from build123d import *

# Parameters (mm, degrees)
F1_DEPTH = 5
F0_W     = 6
F0_H     = 5.5
F0_R     = 1.5
F0_H_2   = 5.75
F2_DEPTH = 25
F4_DEPTH = 105


with BuildPart() as f1:
    # F0 (on Top) → F1 (new body)
    with BuildSketch(Plane.XY):
        Polygon((43.5, 30.25), (-43.5, 30.25), (-43.5, 24.75), (-49.5, 24.75), (-49.5, -24.5), (-43.5, -24.5), (-43.5, -30.25), (43.5, -30.25), (43.5, -24.5), (49.5, -24.5), (49.5, 24.5), (43.5, 24.5), align=None)
    extrude(amount=F1_DEPTH)

    # F0 (on Top) → F2 (join)
    with BuildSketch(Plane.XY):
        with Locations((-46.5, 27.5)):
            Rectangle(F0_W, F0_H)
        with Locations((-46.5, 27.5)):
            Circle(F0_R, mode=Mode.SUBTRACT)
        with Locations((-46.5, -27.375)):
            Rectangle(F0_W, F0_H_2)
        with Locations((-46.5, -27.5)):
            Circle(F0_R, mode=Mode.SUBTRACT)
        with Locations((46.5, -27.375)):
            Rectangle(F0_W, F0_H_2)
        with Locations((46.5, -27.5)):
            Circle(F0_R, mode=Mode.SUBTRACT)
        with Locations((46.5, 27.375)):
            Rectangle(F0_W, F0_H_2)
        with Locations((46.5, 27.5)):
            Circle(F0_R, mode=Mode.SUBTRACT)
    extrude(amount=F2_DEPTH)

    # F3 (on face) → F4 (cut)
    with BuildSketch(Plane.YZ.offset(49.5)):
        Polygon((34.920923, 25), (34.537785, 31.615168), (-33.879854, 31.615168), (-33.879854, 17.220095), align=None)
    extrude(amount=-F4_DEPTH, mode=Mode.SUBTRACT)


solid = f1.part
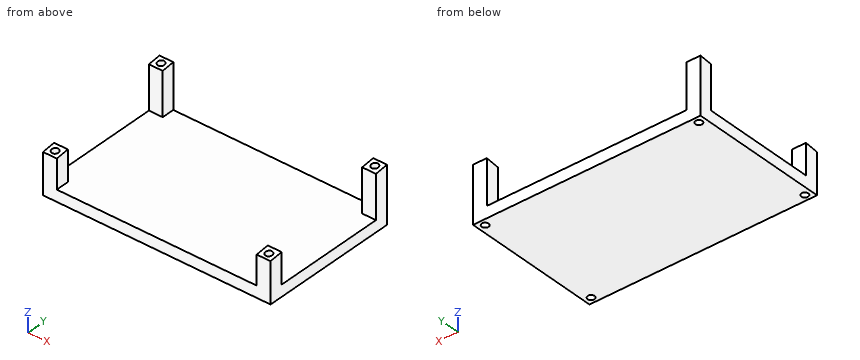
Verification items for the finished model (mm, model axes). Give positions to 0.01 mm unless a question says otherwise; leave off trailing zeros. Loops run counter-clockwise (first coordinate to the right, second up) from the corner with the lowest first, then second, coordinate; pieces in that order, holes last.
1. Cross-section at B-B on z = 8.25. Record the cut outline in (x, y), and give its area (3 significant figures).
Derived:
outline: (-49.5, -30.25) - (-43.5, -30.25) - (-43.5, -24.5) - (-49.5, -24.5) - close; (-49.5, 24.75) - (-43.5, 24.75) - (-43.5, 30.25) - (-49.5, 30.25) - close; (43.5, -30.25) - (49.5, -30.25) - (49.5, -24.5) - (43.5, -24.5) - close; (43.5, 24.5) - (49.5, 24.5) - (49.5, 30.25) - (43.5, 30.25) - close; hole circle Ø3 at (-46.5, -27.5); hole circle Ø3 at (-46.5, 27.5); hole circle Ø3 at (46.5, -27.5); hole circle Ø3 at (46.5, 27.5)
area: 108 mm2
2. Cross-section at C-C on y = -27.5. Record the cut outline in (x, z), and give its area (3 significant figures).
Derived:
outline: (-49.5, 0) - (-48, 0) - (-48, 17.94) - (-49.5, 17.94) - close; (-45, 0) - (45, 0) - (45, 17.94) - (43.5, 17.94) - (43.5, 5) - (-43.5, 5) - (-43.5, 17.94) - (-45, 17.94) - close; (48, 0) - (49.5, 0) - (49.5, 17.94) - (48, 17.94) - close
area: 543 mm2
3. Cross-section at A-A on z = 20.5. Record the cut outline in (x, y), and give its area (3 significant figures).
Derived:
outline: (-49.5, 24.75) - (-43.5, 24.75) - (-43.5, 30.25) - (-49.5, 30.25) - close; (43.5, 24.5) - (49.5, 24.5) - (49.5, 30.25) - (43.5, 30.25) - close; hole circle Ø3 at (-46.5, 27.5); hole circle Ø3 at (46.5, 27.5)
area: 53.4 mm2
4. Material ranges on probe 1 along Y at (x, z) = (-46.5, 9.25); probe 2 along X at (y, z) = (27.5, 11.5); probe 3 along Y at (x, z) = (46.5, 6), recorded low to high.
Derived:
probe 1: y = -30.25 to -29, -26 to -24.5, 24.75 to 26, 29 to 30.25
probe 2: x = -49.5 to -48, -45 to -43.5, 43.5 to 45, 48 to 49.5
probe 3: y = -30.25 to -29, -26 to -24.5, 24.5 to 26, 29 to 30.25
5. Cross-section at D-D on x = -46.5. Record the cut outline in (y, z).
Derived:
outline: (-30.25, 0) - (-29, 0) - (-29, 17.77) - (-30.25, 17.63) - close; (-26, 0) - (26, 0) - (26, 23.99) - (24.75, 23.85) - (24.75, 5) - (-24.5, 5) - (-24.5, 18.28) - (-26, 18.11) - close; (29, 0) - (30.25, 0) - (30.25, 24.47) - (29, 24.33) - close
6. Go/stop test with flat-tipped pins: P1, Ø3.5, axis at x = -46.5, y = -27.5, coming from the +Z side; P2, Ø2.5, axis at x = -46.5, y = 27.5, coming from the -Z side; P3, Ø5, axis at x = 46.5, y = -27.5, coming from the +Z side; P4, Ø5, axis at x = 46.5, y = 27.5, coming from the +Z side. Record where each tip stops, or that it passes through.
Derived:
P1: stops at z = 18.14
P2: passes through
P3: stops at z = 18.22
P4: stops at z = 24.44
